The model under review builds one solid part; all positions refer to its coordinate system, in mm. A direction names the side the tool comes from. Round coordinates to 2 decimals unless told otherwise and drop trailing zeros. Loops run counter-clockwise (first coordinate to the right, second up) from the corner with the lowest first, then second, coordinate; pieces in that order, holes last. Notation, with made-up numbers: (55, 20) -> (77, 20) arc R30 ccw to (77, 56) -> close; hole circle Ø2 at (-13.75, 62.5). An arc over 180 degrees is marked (long way). Write each question's results on one line, items separated by ' | '. Start each with the question number.
Item 1: We need section C-C (y = -1.4). Give the number of separate pieces and of enclosed holes in the cut face, and give its area (3 significant figures).
Item 2: We need section A-A (x = 59.25). Give the boundary of the cut face in (y, z), and give its area (3 significant figures).
Item 3: We need section B-B (z = -59.25). Give the boundary of the cut face in (x, y).
Item 4: Mouldability with a two-part tool opening along X and no side actions: class faces 6 (the cylindrical face through (51.25, 0.01, -46.14)), 7 (the flat face through (-76.2, 0, 9)), 8 (the flat face through (10, 0, -76.2)), 9 (the cylindrical face through (-59.136, -0.398, -61.847)) as pulls with the +X half, pulls with the -X half, needs draft (parallel to the pull), parting line crosses it, or undercut.
Item 5: For L1, parallel to X at y = 0.35, z = 59.25; L2, parallel to X at y = -0.7, z = 59.25; L3, parallel to X at y = -1, z = -59.25, list the stretches that pass through material, from the lowest coordinate up. Write a range as from..to.
Item 6: Clearance check with flat-ended pins moving along their axes: pin 1 Ø1.2 at (y, z) = (1, 74.5) entering from -X; pin 2 Ø2 at (y, z) = (1, -68.5) entering from +X; pin 3 Ø1.2 at (y, z) = (0.5, -73.5) entering from -X; pin 4 Ø8.5 at (x, z) = (-59.25, 59.25) entering from -Y. State where each tip first meets the part, or that it passes through.
Item 7: Tool access review of faces 1 (the cylindrical face through (-46.36, 0.01, 51.25)), 2 (the flat face through (-65, 0, 65.15)), 3 (the flat face through (-71, 0, -46.15)), 4 (the flat face through (76, 0, -35.22)), 5 (the flat face through (4, 2, 4)): name each direction out of +Z, -Z, +X, -X, +Y, -Y from which nothing blocks a thin tool from reaching the whole face with its end or side.
from build123d import *

# Parameters (mm, degrees)
SKETCH1_R           = 1.85
BOSS_EXTRUDE1_DEPTH = 2
CHAMFER2_SIZE       = 1.5
CUT_EXTRUDE2_START  = -2
SKETCH1_4_R         = 2.6
SKETCH1_4_R_2       = 1.85
CUT_EXTRUDE2_DEPTH  = 3.25
FILLET1_R           = 0.75
FILLET2_R           = 1.5


with BuildPart() as part:
    # Sketch1 → Boss-Extrude1 (new, symmetric)
    with BuildSketch(Plane(origin=(0, 0, 0), x_dir=(1, 0, 0), z_dir=(0, 1, 0))):
        with BuildLine():
            Line((-66.2, 46.15), (-76.2, 46.15))
            Line((-76.2, 46.15), (-76.2, -65.15))
            Line((-76.2, -65.15), (-51.25, -65.15))
            Line((-51.25, -65.15), (-51.25, -56.25))
            ThreePointArc((-51.25, -56.25), (-46.25, -51.25), (-41.25, -56.25))
            Line((-41.25, -56.25), (-41.25, -65.15))
            Line((-41.25, -65.15), (-35.22, -65.15))
            Line((-35.22, -65.15), (-35.22, -86.25))
            Line((-35.22, -86.25), (84.75, -86.25))
            ThreePointArc((84.75, -86.25), (85.810660172, -85.810660172), (86.25, -84.75))
            Line((86.25, -84.75), (86.25, 35.22))
            Line((86.25, 35.22), (65.15, 35.22))
            Line((65.15, 35.22), (65.15, 41.25))
            Line((65.15, 41.25), (56.25, 41.25))
            ThreePointArc((56.25, 41.25), (51.25, 46.25), (56.25, 51.25))
            Line((56.25, 51.25), (65.15, 51.25))
            Line((65.15, 51.25), (65.15, 76.2))
            Line((65.15, 76.2), (-46.15, 76.2))
            Line((-46.15, 76.2), (-46.15, 66.2))
            Line((-46.15, 66.2), (-66.2, 66.2))
            Line((-66.2, 66.2), (-66.2, 46.15))
        make_face()
        with Locations(Location((-59.25, 59.25, 0), (0, 0, 270))):
            Circle(SKETCH1_R, mode=Mode.SUBTRACT)
        with Locations(Location((-59.25, -59.25, 0), (0, 0, 270))):
            Circle(SKETCH1_R, mode=Mode.SUBTRACT)
        with Locations(Location((59.25, -59.25, 0), (0, 0, 270))):
            Circle(SKETCH1_R, mode=Mode.SUBTRACT)
        with Locations(Location((59.25, 59.25, 0), (0, 0, 270))):
            Circle(SKETCH1_R, mode=Mode.SUBTRACT)
    extrude(amount=BOSS_EXTRUDE1_DEPTH, both=True)

    # Chamfer2
    chamfer2_edges = [part.edges().sort_by_distance(p)[0] for p in [
        (-59.25, 2, 57.4),
        (59.25, 2, 57.4),
        (59.25, 2, -61.1),
        (-59.25, 2, -61.1),
    ]]
    chamfer(chamfer2_edges, length=CHAMFER2_SIZE)

    # Sketch1<4> → Cut-Extrude2 (cut)
    # profile 1 of 4: a face of its own
    with BuildSketch(Plane(origin=(0, 0, 0), x_dir=(1, 0, 0), z_dir=(0, 1, 0)).offset(CUT_EXTRUDE2_START)):
        with Locations(Location((-59.25, 59.25, 0), (0, 0, 270))):
            Circle(SKETCH1_4_R)
        with Locations((-59.25, 59.25)):
            Circle(SKETCH1_4_R_2, mode=Mode.SUBTRACT)
    # profile 2 of 4: a face of its own
    with BuildSketch(Plane(origin=(0, 0, 0), x_dir=(1, 0, 0), z_dir=(0, 1, 0)).offset(CUT_EXTRUDE2_START)):
        with Locations(Location((-59.25, -59.25, 0), (0, 0, 270))):
            Circle(SKETCH1_4_R)
        with Locations((-59.25, -59.25)):
            Circle(SKETCH1_4_R_2, mode=Mode.SUBTRACT)
    # profile 3 of 4: a face of its own
    with BuildSketch(Plane(origin=(0, 0, 0), x_dir=(1, 0, 0), z_dir=(0, 1, 0)).offset(CUT_EXTRUDE2_START)):
        with Locations(Location((59.25, -59.25, 0), (0, 0, 270))):
            Circle(SKETCH1_4_R)
        with Locations((59.25, -59.25)):
            Circle(SKETCH1_4_R_2, mode=Mode.SUBTRACT)
    # profile 4 of 4: a face of its own
    with BuildSketch(Plane(origin=(0, 0, 0), x_dir=(1, 0, 0), z_dir=(0, 1, 0)).offset(CUT_EXTRUDE2_START)):
        with Locations(Location((59.25, 59.25, 0), (0, 0, 270))):
            Circle(SKETCH1_4_R)
        with Locations((59.25, 59.25)):
            Circle(SKETCH1_4_R_2, mode=Mode.SUBTRACT)
    extrude(amount=CUT_EXTRUDE2_DEPTH, mode=Mode.SUBTRACT)

    # Fillet1
    fillet1_edges = [part.edges().sort_by_distance(p)[0] for p in [
        (24.765, 2, 86.25),
        (85.810660172, 2, 85.810660172),
        (86.25, 2, 24.765),
    ]]
    fillet(fillet1_edges, radius=FILLET1_R)

    # Fillet2
    fillet2_edges = [part.edges().sort_by_distance(p)[0] for p in [
        (51.25, 2, -46.25),
        (60.7, 2, -51.25),
        (-41.25, -2, 60.7),
        (-46.25, -2, 51.25),
        (-51.25, -2, 60.7),
        (60.7, -2, -51.25),
        (51.25, -2, -46.25),
        (60.7, -2, -41.25),
        (65.15, 0, -41.25),
        (-41.25, 0, 65.15),
        (-51.25, 0, 65.15),
        (65.15, 0, -51.25),
        (-51.25, 2, 60.7),
        (-46.25, 2, 51.25),
        (-41.25, 2, 60.7),
        (60.7, 2, -41.25),
    ]]
    fillet(fillet2_edges, radius=FILLET2_R)


solid = part.part
Here are the results:
1) separate pieces: 1 | enclosed holes: 4 | area: 23,800 mm2
2) outline: (-2, -76.2) -> (2, -76.2) -> (2, -62.6) -> (1.25, -61.85) -> (-2, -61.85) -> close; (-2, -56.65) -> (1.25, -56.65) -> (2, -55.9) -> (2, -52.75) arc R1.5 ccw to (0.5, -51.25) -> (-0.5, -51.25) arc R1.5 ccw to (-2, -52.75) -> close; (-2, -39.75) arc R1.5 ccw to (-0.5, -41.25) -> (0.5, -41.25) arc R1.5 ccw to (2, -39.75) -> (2, 55.9) -> (1.25, 56.65) -> (-2, 56.65) -> close; (-2, 61.85) -> (1.25, 61.85) -> (2, 62.6) -> (2, 85.5) arc R0.75 ccw to (1.25, 86.25) -> (-2, 86.25) -> close | area: 565 mm2
3) outline: (-66.2, -2) -> (-61.85, -2) -> (-61.85, 1.25) -> (-62.6, 2) -> (-66.2, 2) -> close; (-56.65, -2) -> (56.65, -2) -> (56.65, 1.25) -> (55.9, 2) -> (-55.9, 2) -> (-56.65, 1.25) -> close; (61.85, -2) -> (65.15, -2) -> (65.15, 2) -> (62.6, 2) -> (61.85, 1.25) -> close
4) face 6: pulls with the +X half | face 7: pulls with the -X half | face 8: needs draft | face 9: undercut
5) L1: x = -76.2..-61.85, -56.65..-51.25, -41.25..56.65, 61.85..86.25 | L2: x = -76.2..-61.85, -56.65..-51.26, -41.24..56.65, 61.85..86.25 | L3: x = -66.2..-61.85, -56.65..56.65, 61.85..65.15
6) pin 1: stops at x = -35.22 | pin 2: stops at x = 65.15 | pin 3: stops at x = -46.15 | pin 4: stops at y = -2
7) face 1: +Z, +Y, -Y | face 2: +Z, -X, +Y, -Y | face 3: -Z, -X, +Y, -Y | face 4: -Z, +X, +Y, -Y | face 5: +Z, -Z, +X, -X, +Y
